Geometry: final body of the model. Coordinates: model frame, mm. A direction names the side the tool comes from. Give positions to 0.01 mm unless a question says otherwise; leave off trailing zeros. Order: outer loops, then holes, each group sorted by start corner. A loop starts at its lowest first (then second) coordinate and runs counter-clockwise, first axis right, second up. Notation, with made-up numbers: (-1, -13) -> (36, -13) arc R22 cw to (36, 8) -> close; hole circle Ø4 at (59, -14.75). An arc over 180 degrees is marked (long way). Write item = value, one per line.
```python
from build123d import *

# Parameters (mm, degrees)
F0_R     = 3.5
F0_R_2   = 1.5
F1_DEPTH = 6
F2_R     = 3.5
F2_R_2   = 1.5
F3_DEPTH = 2
F4_R     = 3.5
F4_R_2   = 3
F5_DEPTH = 2
F4_R_3   = 6
F6_DEPTH = 11
F7_SIZE  = 0.5
F8_SIZE  = 2


with BuildPart() as f1:
    # F0 (on Top) → F1 (new body)
    with BuildSketch(Plane.XY):
        Circle(F0_R)
        Circle(F0_R_2, mode=Mode.SUBTRACT)
    extrude(amount=-F1_DEPTH)

    # F2 (on face) → F3 (join)
    with BuildSketch(Plane.XY):
        Circle(F2_R)
        Circle(F2_R_2, mode=Mode.SUBTRACT)
        Circle(F2_R_2)
    extrude(amount=F3_DEPTH)

    # F4 (on face) → F5 (join)
    with BuildSketch(Plane.XY.offset(2)):
        Circle(F4_R)
        Circle(F4_R_2, mode=Mode.SUBTRACT)
        Circle(F4_R_2)
    extrude(amount=F5_DEPTH)

    # F4 (on face) → F6 (join)
    with BuildSketch(Plane.XY.offset(2)):
        Circle(F4_R_3)
        Circle(F4_R_2, mode=Mode.SUBTRACT)
    extrude(amount=F6_DEPTH)

    # F7
    f7_edges = [f1.edges().sort_by_distance(p)[0] for p in [
        (-3, 0, 13),
        (-6, 0, 13),
        (-1.5, 0, -6),
    ]]
    chamfer(f7_edges, length=F7_SIZE)

    # F8
    f8_edges = [f1.edges().sort_by_distance(p)[0] for p in [
        (-6, 0, 2),
    ]]
    chamfer(f8_edges, length=F8_SIZE)


solid = f1.part
```
1) Mould query, pull axis X, two halves, no side actions, for faces 1 (the face through (0, 0, 4)), 2 (the face through (-6, 0, 8)), 3 (the face through (2, -2, -6)). Classes: +X half, -X half, draft (parallel to the pull), parting line (faces both ways), or undercut.
Check sheet entries:
face_1 = undercut
face_2 = parting line
face_3 = draft
2) First-contact query: P1, Ø3, axis at x = 1.5, y = 0.5, coming from the +Z side; P2, Ø1.5, axis at y = 3.5, z = 10.5, coming from the -X side; P3, Ø6, axis at x = -3.5, z = -3, coming from the -Y side; P4, Ø4, axis at y = 1, z = 9.5, coming from the -X side. Flat tips, straight axial feed; report the tip coordinate or a pass-through.
Check sheet entries:
P1 = 12.58
P2 = -5.33
P3 = -3.46
P4 = -6
3) Reachability of faces 4 (the face through (-1.5, 0.07, -2.71)), 5 (the face through (4, 0, 13)), 6 (the face through (-3, 0, 8)) from +Z, -Z, +X, -X, +Y, -Y: full face, straight path, thin tool, end or side. Return the list, or none.
Check sheet entries:
face_4 = -Z
face_5 = +Z, +X, -X, +Y, -Y
face_6 = +Z
4) Section query A-A (y = 0). Output: boundary loops of the cut face in (x, z), plus the area to 3 significant figures.
Check sheet entries:
outline = (-6, 4) -> (-4, 2) -> (-3.5, 2) -> (-3.5, -6) -> (-2, -6) -> (-1.5, -5.5) -> (-1.5, 0) -> (1.5, 0) -> (1.5, -5.5) -> (2, -6) -> (3.5, -6) -> (3.5, 2) -> (4, 2) -> (6, 4) -> (6, 12.5) -> (5.5, 13) -> (3.5, 13) -> (3, 12.5) -> (3, 4) -> (-3, 4) -> (-3, 12.5) -> (-3.5, 13) -> (-5.5, 13) -> (-6, 12.5) -> close
area = 111 mm²
5) Line query: line 1 (Y direction, x = 0, z = -2.6); line 2 (Z direction, x = 3.75, y = 0); line 3 (Y direction, x = 0, z = 7). Output: solid intervals per line, ascending. Write a range as from..to.
Check sheet entries:
line_1 = -3.5..-1.5, 1.5..3.5
line_2 = 2..13
line_3 = -6..-3, 3..6
6) Section query C-C (z = -5). Output: boundary loops of the cut face in (x, y), plus the area to 3 significant figures.
Check sheet entries:
outline = circle Ø7 at (0, 0); hole circle Ø3 at (0, 0)
area = 31.4 mm²
7) Section query D-D (z = 3.5). Output: boundary loops of the cut face in (x, y), plus the area to 3 significant figures.
Check sheet entries:
outline = circle Ø11 at (0, 0)
area = 95.0 mm²
